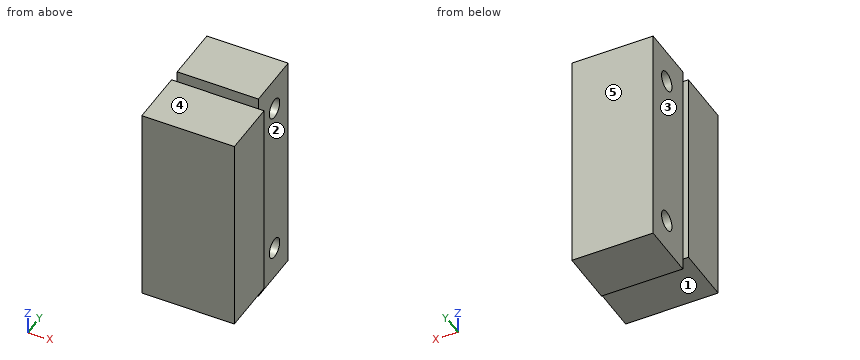
from build123d import *

# Parameters (mm, degrees)
F0_W     = 41.656
F0_H     = 91.44
F1_DEPTH = 25.4
F2_W     = 36.576
F2_H     = 101.6
F3_DEPTH = 25.4
F4_R     = 4.445
F5_DEPTH = 36.576


with BuildPart() as f1:
    # F0 (on Front) → F1 (new body)
    with BuildSketch(Plane.XZ):
        Rectangle(F0_W, F0_H)
    extrude(amount=F1_DEPTH)

    # F2 (on Front) → F3 (join)
    with BuildSketch(Plane.XZ):
        Rectangle(F2_W, F2_H)
    extrude(amount=-F3_DEPTH)

    # F4 (on face) → F5 (cut, through all)
    with BuildSketch(Plane.YZ.offset(18.288)):
        with Locations((13.716, 35.941)):
            Circle(F4_R)
        with Locations((13.716, -35.941)):
            Circle(F4_R)
    extrude(amount=-F5_DEPTH, mode=Mode.SUBTRACT)


solid = f1.part
Could you check a few things on this model? Use its own coordinates, in mm. Face numbers are marked on the shaded views. A direction names the side the tool comes from. Give positions to 0.01 mm unless a question says otherwise; leave off trailing zeros. Loops run counter-clockwise (first coordinate to the right, second up) from the corner with the lowest first, then second, coordinate; pieces in that order, holes last. Notation, with made-up numbers: M 35.25,-26.5 L 48.25,-26.5 A5 ccw 48.25,-18.5 Z; hole C 56.25,16.5 d5. An arc over 180 degrees is marked long. Answer as a JSON object with one key per item and string values.
Q1. Suppose I cut it at C-C, the plane x = 16. List the corners of the cut face in (y, z) for me (3 decimals), plus the area to 3 significant figures.
Values found:
{"outline": "M -25.4,-45.72 L 0,-45.72 L 0,-50.8 L 25.4,-50.8 L 25.4,50.8 L 0,50.8 L 0,45.72 L -25.4,45.72 Z; hole C 13.716,-35.941 d8.89; hole C 13.716,35.941 d8.89", "area": "4,780 mm²"}
Q2. Suppose I cut it at B-B, the plane z = -33. List the corners of the cut face in (x, y) for me, plus the area to 3 significant figures.
Values found:
{"outline": "M -20.83,-25.4 L 20.83,-25.4 L 20.83,0 L 18.29,0 L 18.29,10.38 L -18.29,10.38 L -18.29,0 L -20.83,0 Z; M -18.29,17.05 L 18.29,17.05 L 18.29,25.4 L -18.29,25.4 Z", "area": "1,740 mm²"}
Q3. For the marked faces 1, 2, 3, 4 and 5, which set-ups out of +Z, -Z, +X, -X, +Y, -Y let a thin tool reach every point of the face, with its end or its side?
Values found:
{"face 1": "-Z, +X, -X, -Y", "face 2": "+Z, -Z, +X, +Y", "face 3": "+Z, -Z, -X, +Y", "face 4": "+Z, +X, -X, -Y", "face 5": "+Z, -Z, +X, -X, +Y"}
Q4. Suppose I cut it at D-D, the plane y = -12.5. List the corners of the cut face in (x, z) for me, plus the area to 3 significant figures.
Values found:
{"outline": "M -20.83,-45.72 L 20.83,-45.72 L 20.83,45.72 L -20.83,45.72 Z", "area": "3,810 mm²"}
Q5. If I drill on probe 1 along Z at (x, y) = (11, 12.5); probe 2 along Z at (x, y) = (5.5, 14); probe 3 along Y at (x, z) = (10, -35.5), over which ranges is the centre line in solid material (lowest first)? Write a range as [from, to].
Values found:
{"probe 1": "z = [-50.8, -40.22], [-31.67, 31.67], [40.22, 50.8]", "probe 2": "z = [-50.8, -40.38], [-31.51, 31.51], [40.38, 50.8]", "probe 3": "y = [-25.4, 9.29], [18.14, 25.4]"}
Q6. Suppose I cut it at A-A, the plane y = 14. List the corners of the cut face in (x, z) for me.
Values found:
{"outline": "M -18.29,-50.8 L 18.29,-50.8 L 18.29,-40.38 L -18.29,-40.38 Z; M -18.29,-31.51 L 18.29,-31.51 L 18.29,31.51 L -18.29,31.51 Z; M -18.29,40.38 L 18.29,40.38 L 18.29,50.8 L -18.29,50.8 Z"}
Q7. For P1, Ø2, axis at x = -1, y = -18, coming from the +Z side; P2, Ø20.5, axis at x = -5, y = -14, coming from the -Z side; P3, Ø2.5, axis at x = 5.5, z = -48, coming from the -Y side, each with a flat end and sliding along its axis, tell me the tip position at first contact or that it passes through.
Values found:
{"P1": "stops at z = 45.72", "P2": "stops at z = -45.72", "P3": "stops at y = 0"}
